```python
from build123d import *

# Parameters (mm, degrees)
F0_W     = 304.8
F0_H     = 152.4
F1_DEPTH = 304.8
F3_DEPTH = 5
F4_W     = 19.05
F4_H     = 50.8
F5_DEPTH = 2.5


with BuildPart() as f1:
    # F0 (on Top) → F1 (new body)
    with BuildSketch(Plane.XY):
        with Locations((-2.632114, -74.741666)):
            Rectangle(F0_W, F0_H)
    extrude(amount=F1_DEPTH)

    # F2 (on face) → F3 (join)
    with BuildSketch(Plane.XZ.offset(150.941666)):
        Polygon((-7.632114, 304.8), (-155.032114, 304.8), (-155.032114, 0), (-7.632114, 0), (-7.632114, 5), (-7.632114, 299.8), align=None)
        Polygon((149.767886, 304.8), (2.367886, 304.8), (2.367886, 299.8), (2.367886, 5), (2.367886, 0), (149.767886, 0), align=None)
    extrude(amount=F3_DEPTH)

    # F4 (on face) → F5 (join)
    with BuildSketch(Plane.XZ.offset(155.941666)):
        with Locations((-130.563368, 249.110587)):
            Rectangle(F4_W, F4_H)
    extrude(amount=F5_DEPTH)


solid = f1.part
```
Source: CAD feature listing. Evaluate the final solid. Frame: model axes, mm. A direction names the side the tool comes from. Round coordinates to 2 decimals unless told otherwise and drop trailing zeros. Loops run counter-clockwise (first coordinate to the right, second up) from the corner with the lowest first, then second, coordinate; pieces in that order, holes last. Notation, with made-up numbers: M 6.25,-5.5 L 13.25,-5.5 A21 cw 13.25,27.5 Z; hole C 33,79 d2. An arc over 180 degrees is marked long. Use a Markdown table: item, result. Add a question column.
1. Section query C-C on z = 255. Return the cut outline in (x, y), then the cut area to 3 significant figures.
2. Line query: line 1 (Y direction, x = -83, z = 179); line 2 (Y direction, x = -5, z = 111). Output: solid intervals per line, ascending.
3. Section query A-A on z = 183. Return the cut outline in (x, y), then the cut area to 3 significant figures.
4. Section query B-B on x = -40. Return the cut outline in (y, z).
5. Contact query for flat-ended pins moving along their axis: P1, Ø2, axis at y = -156.5, z = 253, coming from the +X side; P2, Ø11, axis at x = -1.5, z = 158, coming from the -Y side; P3, Ø0.8, axis at x = -127, y = -157.5, coming from the -Z side; P4, Ø2, axis at x = -135, y = -157, coming from the +Z side. Output: stop coordinate, or through.
6. Reachability of faces 1 (the flat face through (-3, -150.942, 150)), 2 (the flat face through (0, -76, 304.8)) from +Z, -Z, +X, -X, +Y, -Y: full face, straight path, thin tool, end or side. Return the list, or none.
Reported:
| question | item | result |
|---|---|---|
| 1 | outline | M -155.03,-155.94 L -140.09,-155.94 L -140.09,-158.44 L -121.04,-158.44 L -121.04,-155.94 L -7.63,-155.94 L -7.63,-150.94 L 2.37,-150.94 L 2.37,-155.94 L 149.77,-155.94 L 149.77,1.46 L -155.03,1.46 Z |
| 1 | area | 48,000 mm² |
| 2 | line 1 | y = -155.94 to 1.46 |
| 2 | line 2 | y = -150.94 to 1.46 |
| 3 | outline | M -155.03,-155.94 L -7.63,-155.94 L -7.63,-150.94 L 2.37,-150.94 L 2.37,-155.94 L 149.77,-155.94 L 149.77,1.46 L -155.03,1.46 Z |
| 3 | area | 47,900 mm² |
| 4 | outline | M -155.94,0 L 1.46,0 L 1.46,304.8 L -155.94,304.8 Z |
| 5 | P1 | stops at x = 149.77 |
| 5 | P2 | stops at y = -155.94 |
| 5 | P3 | stops at z = 223.71 |
| 5 | P4 | stops at z = 274.51 |
| 6 | face 1 | +Z, -Z, -Y |
| 6 | face 2 | +Z, +X, -X, +Y, -Y |
